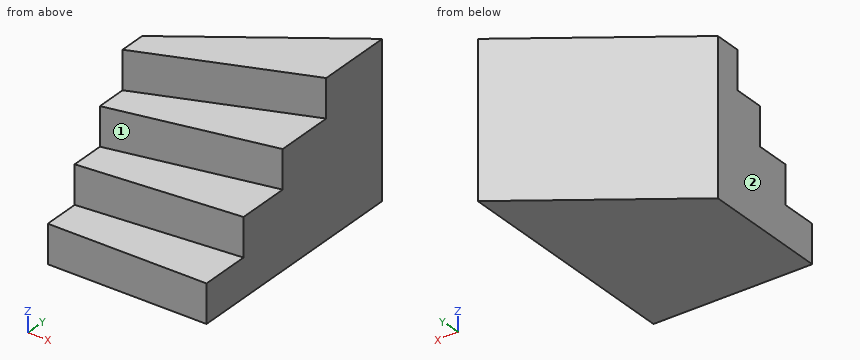
```python
from build123d import *

# Parameters (mm, degrees)
F1_DEPTH = 192
F2_DEPTH = 384
F3_DEPTH = 576
F4_DEPTH = 768


with BuildPart() as f1:
    # F0 (on Top) → F1 (new body)
    with BuildSketch(Plane.XY):
        Polygon((1188.775452454, -1224.3236021269), (1188.775452454, -970.2663376007), (388.775452454, -1039.3673186817), (388.775452454, -1224.3236021269), align=None)
    extrude(amount=F1_DEPTH)

    # F0 (on Top) → F2 (join)
    with BuildSketch(Plane.XY):
        Polygon((1188.775452454, -970.2663376007), (1188.775452454, -701.3968009689), (388.775452454, -866.2996554468), (388.775452454, -1039.3673186817), align=None)
    extrude(amount=F2_DEPTH)

    # F0 (on Top) → F3 (join)
    with BuildSketch(Plane.XY):
        Polygon((1188.775452454, -701.3968009689), (1188.775452454, -402.0830337411), (388.775452454, -710.5429181553), (388.775452454, -866.2996554468), align=None)
    extrude(amount=F3_DEPTH)

    # F0 (on Top) → F4 (join)
    with BuildSketch(Plane.XY):
        Polygon((1188.775452454, -402.0830337411), (1188.775452454, -17.5821596523), (735.1856139678, -334.3236021269), (448.775452454, -534.3236021269), (388.775452454, -576.2215569221), (388.775452454, -710.5429181553), align=None)
    extrude(amount=F4_DEPTH)


solid = f1.part
```
Geometry: final body of the model. Coordinates: model frame, mm. Face numbers are marked on the shaded views. A direction names the side the tool comes from. Round coordinates to 2 decimals unless told otherwise and drop trailing zeros. Order: outer loops, then holes, each group sorted by start corner. A loop starts at its lowest first (then second) coordinate and runs counter-clockwise, first axis right, second up. Notation, with made-up numbers: (61.5, 57) -> (116.5, 57) arc R25 ccw to (116.5, 86) -> close; hole circle Ø6 at (37, 50.25). An arc over 180 degrees is marked (long way). Use CSV: the item, a comma, the result in double quotes. Start each with the question number.
1) Material intervals for line 1 along Z through (x, y) = (1002.5, -530); line 2 along Z through (x, y) = (1148, -859); line 3 along Y through (x, z) = (607, 616.5), sorted ascending. Write a range as from..to.
2) Section B-B (y = -613.5). Return the cut outline in (x, z).
3) First-contact query: pin 1 Ø1 at (x, z) = (741.5, 320) entering from -Y; pin 2 Ø3 at (x, y) = (648.5, -438) entering from -Z; pin 3 Ø12 at (x, z) = (783.5, 321.5) entering from -Y; pin 4 Ø1 at (x, z) = (485, 472.5) entering from -Y. Flat tips, straight axial feed; report the tip coordinate or a pass-through.
4) Section D-D (x = 789). Return the cut outline in (y, z), and give its area (3 significant figures).
5) Set-up query: the marked faces 1 and 2. Return all of +Z, -Z, +X, -X, +Y, -Y with unobstructed straight access to the full face (end or side cutting, diameter ignored); none if empty.
6) Section C-C (z = 129). Return the cut outline in (x, y), and give its area (3 significant figures).
7) Section A-A (x = 484). Return the cut outline in (y, z).
Returned:
1,line 1,"z = 0..576"
1,line 2,"z = 0..384"
1,line 3,"y = -626.4..-423.84"
2,outline,"(388.78, 0) -> (1188.78, 0) -> (1188.78, 576) -> (640.46, 576) -> (640.46, 768) -> (388.78, 768) -> close"
3,pin 1,"stops at y = -1008.94"
3,pin 2,"stops at z = 0"
3,pin 3,"stops at y = -1005.79"
3,pin 4,"stops at y = -846.57"
4,outline,"(-1224.32, 0) -> (-296.75, 0) -> (-296.75, 768) -> (-556.23, 768) -> (-556.23, 576) -> (-783.8, 576) -> (-783.8, 384) -> (-1004.8, 384) -> (-1004.8, 192) -> (-1224.32, 192) -> close"
4,area,"457,000 mm²"
5,face 1,"+Z, +X, -Y"
5,face 2,"+Z, -Z, -X, +Y, -Y"
6,outline,"(388.78, -1224.32) -> (1188.78, -1224.32) -> (1188.78, -17.58) -> (388.78, -576.22) -> close"
6,area,"742,000 mm²"
7,outline,"(-1224.32, 0) -> (-509.73, 0) -> (-509.73, 768) -> (-673.83, 768) -> (-673.83, 576) -> (-846.67, 576) -> (-846.67, 384) -> (-1031.14, 384) -> (-1031.14, 192) -> (-1224.32, 192) -> close"
